```python
from build123d import *

# Parameters (mm, degrees)
SKETCH1_R           = 1
BOSS_EXTRUDE1_DEPTH = 3
SKETCH2_R           = 27.5
SKETCH2_R_2         = 1
CUT_EXTRUDE1_DEPTH  = 3


with BuildPart() as part:
    # Sketch1 → Boss-Extrude1 (new body)
    with BuildSketch(Plane.YZ):
        Polygon((-80, 60), (-80, 65), (-60, 65), (-60, 60), (-10, 60), (-10, 65), (10, 65), (10, 60), (60, 60), (60, 65), (80, 65), (80, 60), (100, 60), (100, -60), (80, -60), (80, -65), (60, -65), (60, -60), (10, -60), (10, -65), (-10, -65), (-10, -60), (-60, -60), (-60, -65), (-80, -65), (-80, -60), (-100, -60), (-100, 60), align=None)
        with Locations(Location((-70, 61, 0), (0, 0, 270))):
            Circle(SKETCH1_R, mode=Mode.SUBTRACT)
        with Locations(Location((70, 61, 0), (0, 0, 270))):
            Circle(SKETCH1_R, mode=Mode.SUBTRACT)
        with Locations(Location((0, 61, 0), (0, 0, 270))):
            Circle(SKETCH1_R, mode=Mode.SUBTRACT)
        with Locations(Location((70, -61, 0), (0, 0, 270))):
            Circle(SKETCH1_R, mode=Mode.SUBTRACT)
        with Locations(Location((0, -61, 0), (0, 0, 270))):
            Circle(SKETCH1_R, mode=Mode.SUBTRACT)
        with Locations(Location((-70, -61, 0), (0, 0, 270))):
            Circle(SKETCH1_R, mode=Mode.SUBTRACT)
    extrude(amount=BOSS_EXTRUDE1_DEPTH)

    # Sketch2 → Cut-Extrude1 (cut)
    with BuildSketch(Plane.YZ.offset(3)):
        with Locations(Location((0, 0, 0), (0, 0, 270))):
            Circle(SKETCH2_R)
        with Locations(Location((72.5, -12.5, 0), (0, 0, 270))):
            Circle(SKETCH2_R_2)
        with Locations(Location((72.5, 12.5, 0), (0, 0, 90))):
            Circle(SKETCH2_R_2)
        with BuildLine():
            Line((67.527461624, 8.686817334), (67.527461624, -8.686817334))
            ThreePointArc((67.527461624, -8.686817334), (64.996283302, -11.217995655), (62.465104981, -8.686817334))
            Line((62.465104981, -8.686817334), (62.465104981, 8.686817334))
            ThreePointArc((62.465104981, 8.686817334), (64.996283302, 11.217995655), (67.527461624, 8.686817334))
        make_face()
    extrude(amount=-CUT_EXTRUDE1_DEPTH, mode=Mode.SUBTRACT)


solid = part.part
```
Can you work these out from the model? Positions are in its coordinate system, mm. Give positions to 0.01 mm unless a question says otherwise; leave off trailing zeros. Loops run counter-clockwise (first coordinate to the right, second up) from the corner with the lowest first, then second, coordinate; pieces in that order, holes last. Notation, with made-up numbers: M 64.25,-37.75 L 108.25,-37.75 A20 ccw 108.25,-5.75 Z; hole C -9,37 d10. An arc over 180 degrees is marked long. Use one line per item in the form item = value. Start each with the question number.
(1) I want a section at B-B, the plane y = 12.5. Write out the boundary of the cut face in (x, z), and give its area (3 significant figures).
(2) Please list where these lines run through material, in increasing order: line 1 (Y direction, x = 1.2, z = -61); line 2 (Z direction, x = 1.7, y = 70); line 3 (Z direction, x = 1.05, y = 72.5).
(3) I want a section at A-A, the plane z = 25. Write out the boundary of the cut face in (x, y).
(4) I want a section at D-D, the plane x = 0.6. State how many separate pieces and enclosed holes the cut face has, and give its area (3 significant figures).
(5) I'm going to push flat-ended pins straight in: P1, Ø0.9, axis at x = 1, z = -61.5, coming from the -Y side; P2, Ø0.9, axis at x = 1, y = -28.5, coming from the +Z side; P3, Ø1.5, axis at x = 2, z = -62.5, coming from the +Y side. Where does each tip first touch, or does it pass through?
(6) Thinking about a two-plate mould opening in Z: for faces 1 (the cylindrical face through (1.521, -24.397, -12.69)), 2 (the flat face through (3, 24, 15)), which applies, released by +Z, released by -Z, zero draft, split by the parting line, or undercut?
(7) I want a section at C-C, the plane y = -83.5. Write out the boundary of the cut face in (x, z), and give its area (3 significant figures).
Worked out:
q1.outline = M 0,-60 L 3,-60 L 3,-24.49 L 0,-24.49 Z; M 0,24.49 L 3,24.49 L 3,60 L 0,60 Z
q1.area = 213 mm²
q2.line_1 = -80 to -71, -69 to -60, -10 to -1, 1 to 10, 60 to 69, 71 to 80
q2.line_2 = -65 to -62, -60 to 60, 62 to 65
q2.line_3 = -65 to -13.5, -11.5 to 11.5, 13.5 to 65
q3.outline = M 0,-100 L 3,-100 L 3,-11.46 L 0,-11.46 Z; M 0,11.46 L 3,11.46 L 3,100 L 0,100 Z
q4.separate_pieces = 1
q4.enclosed_holes = 10
q4.area = 22,100 mm²
q5.P1 = -80
q5.P2 = 60
q5.P3 = 80
q6.face_1 = undercut
q6.face_2 = zero draft
q7.outline = M 0,-60 L 3,-60 L 3,60 L 0,60 Z
q7.area = 360 mm²
